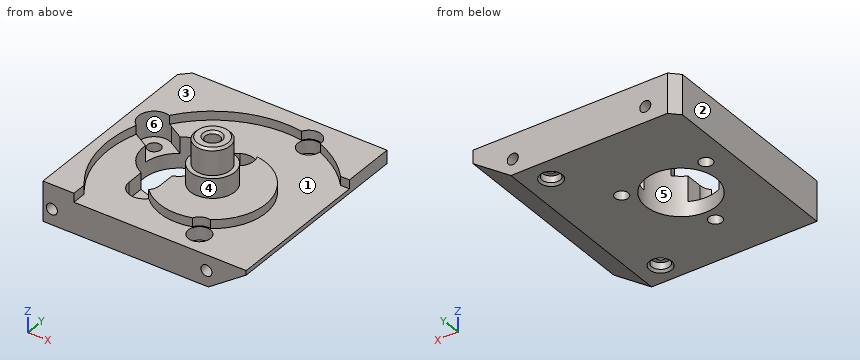
from build123d import *

# Parameters (mm, degrees)
SKETCH_1_W                  = 52
SKETCH_1_H                  = 47
EXTRUDE_1_DEPTH             = 9
SKETCH_19_R                 = 23.75
SKETCH_19_R_2               = 12
CUT_EXTRUDE_2_DEPTH         = 2
SKETCH_20_R                 = 5
EXTRUDE_3_DEPTH             = 4.4
SKETCH_21_R                 = 4
EXTRUDE_4_DEPTH             = 6
SKETCH_22_R                 = 8
CUT_EXTRUDE_5_DEPTH         = 37.556941885
CUT_EXTRUDE_6_DEPTH         = 47
HOLE_WIZARD_M3_1_D          = 2.5
HOLE_WIZARD_M3_1_DEPTH      = 9.5
HOLE_WIZARD_M3_1_TIP        = 0.751075774
HOLE_WIZARD_M4_2_D          = 3.3
HOLE_WIZARD_M4_2_DEPTH      = 10.1
HOLE_WIZARD_M4_2_TIP        = 0.991420021
CHAMFER_3_SIZE              = 0.5
CHAMFER_5_SIZE              = 2
EXTRUDE3_DEPTH              = 2
EXTRUDE4_REACH              = 57.474
CUT_EXTRUDE_START           = -31
SKETCH_34_R                 = 8
CUT_EXTRUDE_1_DEPTH         = 31
SKETCH_35_R                 = 3.25
CUT_EXTRUDE_2_2_DEPTH       = 33
PATTERN_CIRCULAR_1_COUNT    = 3
HOLE_WIZARD_2_AT_2_COUNT    = 2
HOLE_WIZARD_2_AT_2_PITCH    = 19.052558883
HOLE_WIZARD_2_AT_3_COUNT    = 2
HOLE_WIZARD_2_AT_3_PITCH    = 19.052558883
HOLE_WIZARD_M3_2_D          = 2.5
HOLE_WIZARD_M3_2_DEPTH      = 9.5
HOLE_WIZARD_M3_2_TIP        = 0.751075774
SKETCH_39_R                 = 2
CUT_EXTRUDE_3_DEPTH         = 2
SKETCH_40_R                 = 2.75
CUT_EXTRUDE_4_DEPTH         = 2
SKETCH_41_R                 = 1.1
CUT_EXTRUDE_5_2_DEPTH       = 37
CHAMFER_7_SIZE              = 0.5
HOLE_WIZARD_2_2_D           = 2
HOLE_WIZARD_2_2_CBORE_D     = 5
HOLE_WIZARD_2_2_CBORE_DEPTH = 3
CUT_EXTRUDE_START_2         = 7
CUT_EXTRUDE_7_DEPTH         = 7
PATTERN_CIRCULAR_2_COUNT    = 3
SKETCH_45_W                 = 2.943459277
SKETCH_45_H                 = 3.25
SKETCH_45_W_2               = 2.005209087
SKETCH_45_H_2               = 2.691311543
SKETCH_45_W_3               = 3.943459277
SKETCH_45_H_3               = 4.763787499
CUT_EXTRUDE_8_DEPTH         = 2


with BuildPart() as part:
    # 草图1 → 拉伸1 (new body)
    with BuildSketch(Plane.XY):
        Rectangle(SKETCH_1_W, SKETCH_1_H)
    extrude(amount=EXTRUDE_1_DEPTH)

    # 草图19 → Cut-Extrude 2 (cut)
    with BuildSketch(Plane.XY.offset(9)):
        with Locations((0, -4)):
            Circle(SKETCH_19_R)
        with Locations((0, -4)):
            Circle(SKETCH_19_R_2, mode=Mode.SUBTRACT)
    extrude(amount=-CUT_EXTRUDE_2_DEPTH, mode=Mode.SUBTRACT)

    # 草图20 → 拉伸3 (add)
    with BuildSketch(Plane.XY.offset(9)):
        with Locations((0, -4)):
            Circle(SKETCH_20_R)
    extrude(amount=EXTRUDE_3_DEPTH)

    # 草图21 → 拉伸4 (add)
    with BuildSketch(Plane.XY.offset(13.4)):
        with Locations((0, -4)):
            Circle(SKETCH_21_R)
    extrude(amount=EXTRUDE_4_DEPTH)

    # 草图22 → Cut-Extrude 5 (cut, through all)
    with BuildSketch(Plane.XY.offset(9)):
        with Locations((-11, 0.795831523)):
            Circle(SKETCH_22_R)
    extrude(amount=-CUT_EXTRUDE_5_DEPTH, mode=Mode.SUBTRACT)

    # 草图25 → 拉伸6 (cut)
    with BuildSketch(Plane.XZ.offset(23.5)):
        Polygon((26, 8), (14.574815946, 0), (26, 0), align=None)
    extrude(amount=-CUT_EXTRUDE_6_DEPTH, mode=Mode.SUBTRACT)

    # M3 螺纹孔1
    with Locations(Plane(origin=(11, 23.5, 3.5), x_dir=(0, 0, 1), z_dir=(0, 1, 0))):
        with Locations((0, 0), (0, -30)):
            Hole(HOLE_WIZARD_M3_1_D / 2, depth=HOLE_WIZARD_M3_1_DEPTH)
            with Locations((0, 0, -(HOLE_WIZARD_M3_1_DEPTH + HOLE_WIZARD_M3_1_TIP / 2))):  # 118° drill point
                Cone(0, HOLE_WIZARD_M3_1_D / 2, HOLE_WIZARD_M3_1_TIP, mode=Mode.SUBTRACT)

    # M4 螺纹孔2
    with Locations(Plane(origin=(0, -4, 19.4), x_dir=(1, 0, 0), z_dir=(0, 0, 1))):
        with Locations((0, 0)):
            Hole(HOLE_WIZARD_M4_2_D / 2, depth=HOLE_WIZARD_M4_2_DEPTH)
            with Locations((0, 0, -(HOLE_WIZARD_M4_2_DEPTH + HOLE_WIZARD_M4_2_TIP / 2))):  # 118° drill point
                Cone(0, HOLE_WIZARD_M4_2_D / 2, HOLE_WIZARD_M4_2_TIP, mode=Mode.SUBTRACT)

    # 倒角3
    chamfer_3_edges = [part.edges().sort_by_distance(p)[0] for p in [
        (-4, -4, 19.4),
        (1.65, -4, 19.4),
    ]]
    chamfer(chamfer_3_edges, length=CHAMFER_3_SIZE)

    # 倒角5
    chamfer_5_edges = [part.edges().sort_by_distance(p)[0] for p in [
        (-26, 23.5, 4.5),
    ]]
    chamfer(chamfer_5_edges, length=CHAMFER_5_SIZE)

    # Sketch4 → Extrude3 (cut)
    with BuildSketch(Plane.XZ.offset(23.5)):
        Polygon((-26, 0), (14.574815946, 0), (26, 8), (26, 9), (13.557746863, 9), (13.557746863, 7), (-13.557746863, 7), (-13.557746863, 9), (-26, 9), align=None)
    extrude(amount=-EXTRUDE3_DEPTH, mode=Mode.SUBTRACT)

    # Extrude4: up to this face of the body (flat: up to its plane)
    extrude4_end = Plane(part.part.faces().sort_by_distance((-1.330613504, 23.5, 4.737278788))[0])
    # Sketch5 → Extrude4 (cut, up to the picked face)
    with BuildSketch(Plane.XZ.offset(21.5), mode=Mode.PRIVATE) as extrude4_sk1:
        Polygon((26, 9), (20, 9), (20, 6), (11.43111196, 0), (14.574815946, 0), (26, 8), align=None)
    extrude4_tool1 = split(extrude(extrude4_sk1.sketch, amount=-EXTRUDE4_REACH, mode=Mode.PRIVATE), bisect_by=extrude4_end, keep=Keep.BOTH, mode=Mode.PRIVATE)
    add(extrude4_tool1.solids().sort_by(Axis((19.659359, -21.5, 5.073959), (0, 1, 0)))[0], mode=Mode.SUBTRACT)

    # 草图34 → 切除-拉伸1 (cut)
    with BuildSketch(Plane(origin=(0, 0, 0), x_dir=(-1, 0, 0), z_dir=(0, 0, -1)).offset(CUT_EXTRUDE_START)):
        with Locations(Location((11, 0.795831523, 0), (0, 0, 180))):
            Circle(SKETCH_34_R)
    extrude(amount=CUT_EXTRUDE_1_DEPTH, mode=Mode.SUBTRACT)

    # 草图35 → Cut-Extrude 2 2 (cut)
    with BuildSketch(Plane.XY.offset(7)):
        with Locations((-1.473720558, 6.295831523)):
            Circle(SKETCH_35_R)
    cut_extrude_2_2 = extrude(amount=CUT_EXTRUDE_2_2_DEPTH, mode=Mode.SUBTRACT)

    # 阵列(圆周)1: Cut-Extrude 2 2 ×3 about axis
    pattern_circular_1_axis = Axis((-11, 0.795831523, 0), (0, 0, 1))
    for i in range(1, PATTERN_CIRCULAR_1_COUNT):
        add(cut_extrude_2_2.rotate(pattern_circular_1_axis, i * 360 / PATTERN_CIRCULAR_1_COUNT), mode=Mode.SUBTRACT)

    # 草图36 → Hole Wizard 2 (revolve, cut)
    with BuildSketch(Plane(origin=(-20.526279442, 6.295831523, 7), x_dir=(0, -1, 0), z_dir=(1, 0, 0))):
        Polygon((0, 0), (0, 7), (1.5, 7), (1.5, 3.7), (3.5, 3.7), (3.5, 0), align=None)
    hole_wizard_2 = revolve(axis=Axis((-20.526279442, 6.295831523, 13.35), (0, 0, -1)), mode=Mode.SUBTRACT)

    # Hole Wizard 2 at 2: Hole Wizard 2 ×2
    with Locations(*[(i * HOLE_WIZARD_2_AT_2_PITCH, 0, 0) for i in range(1, HOLE_WIZARD_2_AT_2_COUNT)]):
        add(hole_wizard_2, mode=Mode.SUBTRACT)

    # Hole Wizard 2 at 3: Hole Wizard 2 ×2
    with Locations(*[Vector(0.49999999999999795, -0.8660254037844398, 0) * (i * HOLE_WIZARD_2_AT_3_PITCH) for i in range(1, HOLE_WIZARD_2_AT_3_COUNT)]):
        add(hole_wizard_2, mode=Mode.SUBTRACT)

    # M3 螺纹孔2
    with Locations(Plane(origin=(-24, -21.5, 3.5), x_dir=(0, 0, -1), z_dir=(0, -1, 0))):
        with Locations((0, 0), (0, 35)):
            Hole(HOLE_WIZARD_M3_2_D / 2, depth=HOLE_WIZARD_M3_2_DEPTH)
            with Locations((0, 0, -(HOLE_WIZARD_M3_2_DEPTH + HOLE_WIZARD_M3_2_TIP / 2))):  # 118° drill point
                Cone(0, HOLE_WIZARD_M3_2_D / 2, HOLE_WIZARD_M3_2_TIP, mode=Mode.SUBTRACT)

    # 草图39 → 切除-拉伸3 (cut)
    with BuildSketch(Plane(origin=(0, 0, 0), x_dir=(-1, 0, 0), z_dir=(0, 0, -1))):
        with Locations((-6, 18.295831523)):
            Circle(SKETCH_39_R)
        with Locations((-6, -16.704168477)):
            Circle(SKETCH_39_R)
    extrude(amount=-CUT_EXTRUDE_3_DEPTH, mode=Mode.SUBTRACT)

    # 草图40 → 切除-拉伸4 (cut)
    with BuildSketch(Plane.XY.offset(9)):
        with Locations((6, 18.295831523)):
            Circle(SKETCH_40_R)
        with Locations((6, -16.704168477)):
            Circle(SKETCH_40_R)
    extrude(amount=-CUT_EXTRUDE_4_DEPTH, mode=Mode.SUBTRACT)

    # 草图41 → Cut-Extrude 5 2 (cut)
    with BuildSketch(Plane(origin=(0, 0, 2), x_dir=(-1, 0, 0), z_dir=(0, 0, -1))):
        with Locations((-6, 18.295831523)):
            Circle(SKETCH_41_R)
        with Locations((-6, -16.704168477)):
            Circle(SKETCH_41_R)
    extrude(amount=-CUT_EXTRUDE_5_2_DEPTH, mode=Mode.SUBTRACT)

    # 倒角7
    chamfer_7_edges = [part.edges().sort_by_distance(p)[0] for p in [
        (8, 18.295831523, 0),
        (8, -16.704168477, 0),
    ]]
    chamfer(chamfer_7_edges, length=CHAMFER_7_SIZE)

    # Hole Wizard 2 2 (through all)
    with Locations(Plane(origin=(6, 18.295831523, 7), x_dir=(1, 0, 0), z_dir=(0, 0, 1))):
        with Locations((0, 0), (0, -35)):
            CounterBoreHole(HOLE_WIZARD_2_2_D / 2, HOLE_WIZARD_2_2_CBORE_D / 2, HOLE_WIZARD_2_2_CBORE_DEPTH)

    # 草图44 → 切除-拉伸7 (cut)
    with BuildSketch(Plane.XY.offset(3.3).offset(CUT_EXTRUDE_START_2)):
        with BuildLine():
            Line((0.276279442, 3.26474261), (-9.25, -2.23525739))
            ThreePointArc((-9.25, -2.23525739), (-14.031088913, -0.954168477), (-12.75, 3.826920437))
            Line((-12.75, 3.826920437), (-3.223720558, 9.326920437))
            ThreePointArc((-3.223720558, 9.326920437), (1.557368355, 8.045831523), (0.276279442, 3.26474261))
        make_face()
    cut_extrude_7 = extrude(amount=-CUT_EXTRUDE_7_DEPTH, mode=Mode.SUBTRACT)

    # 阵列(圆周)2: 切除-拉伸7 ×3 about axis
    pattern_circular_2_axis = Axis((-11, 0.795831523, 0), (0, 0, 1))
    for i in range(1, PATTERN_CIRCULAR_2_COUNT):
        add(cut_extrude_7.rotate(pattern_circular_2_axis, i * 360 / PATTERN_CIRCULAR_2_COUNT), mode=Mode.SUBTRACT)

    # 草图45 → 切除-拉伸8 (cut)
    with BuildSketch(Plane.XY.offset(9)):
        with Locations((-17.528270361, -19.875)):
            Rectangle(SKETCH_45_W, SKETCH_45_H)
        with Locations((18.997395457, 10.154344229)):
            Rectangle(SKETCH_45_W_2, SKETCH_45_H_2)
        with Locations((18.028270361, -19.11810625)):
            Rectangle(SKETCH_45_W_3, SKETCH_45_H_3)
    extrude(amount=-CUT_EXTRUDE_8_DEPTH, mode=Mode.SUBTRACT)


solid = part.part
Design review of the part built by this model. Coordinates are the model's own, in mm. Face numbers are marked on the shaded views. A direction names the side the tool comes from. Coordinates: 2 decimals unless noted, no trailing zeros. Loops run counter-clockwise (first coordinate to the right, second up) from the corner with the lowest first, then second, coordinate; pieces in that order, holes last.
Item 1: Clearance check with flat-ended pins moving along their axes: pin 1 (2.5 mm diameter, centred on x = 7, y = -18, fed in from +Z); pin 2 (1.5 mm diameter, centred on y = -5.5, z = 10, fed in from +X); pin 3 (2.5 mm diameter, centred on x = 6, y = -16.7, fed in from -Z). State where each tip first meets the part, or that it passes through.
Completed:
pin 1: stops at z = 7
pin 2: stops at x = 4.94
pin 3: stops at z = 2
Item 2: Add section B-B (x = -11). Write out the cut boundary in (y, z).
Completed:
outline: (-21.5, 0) - (-11.7, 0) - (-11.7, 3.3) - (-13.7, 3.3) - (-13.7, 7) - (-21.5, 7) - close; (-8.7, 0) - (-7.2, 0) - (-7.2, 3.3) - (-8.7, 3.3) - close; (8.8, 0) - (23.5, 0) - (23.5, 9) - (17.05, 9) - (17.05, 7) - (8.8, 7) - close
Item 3: Wall thickness on L1, parallel to Y at x = 6, z = 4.6; L2, parallel to Y at x = 6, z = 0.85; L3, parallel to Z at x = 11, y = -16: over which ranges is each line inside the solid? List them lowest first.
Completed:
L1: y = -21.5 to -19.2, -14.2 to 15.8, 20.8 to 23.5
L2: y = -21.5 to -18.7, -14.7 to 16.3, 20.3 to 23.5
L3: z = 0 to 2.25, 4.75 to 7
Item 4: Add section C-C (z = 18.25). Write out the cut boundary in (x, y).
Completed:
outline: circle Ø8 at (0, -4); hole circle Ø3.3 at (0, -4)
Item 5: For the marked faces 5 and 6, list the 3-axis set-ups (+Z, -Z, +X, -X, +Y, -Y) from which the entire face can be reached by the end or side of a thin tool; tool diameter is ignored.
Completed:
face 5: +Z, -Z
face 6: +Z
Item 6: Draft analysis for pull direction X (two halves, no side actions). For the marked faces 1, 2, 3 and 4, state which applies: pulls with the +X half, pulls with the -X half, needs draft (parallel to the pull), parting line crosses it, or undercut.
Completed:
face 1: undercut
face 2: pulls with the -X half
face 3: needs draft
face 4: parting line crosses it
Item 7: Add section D-D (x = 6). Give the number of separate pieces and of enclosed holes in the cut face, and give its area (3 significant figures).
Completed:
separate pieces: 3
enclosed holes: 0
area: 305 mm2
Item 8: Add section A-A (y = 6). Write out the cut boundary in (x, z).
Completed:
outline: (-26, 0) - (-22, 0) - (-22, 3.3) - (-24.01, 3.3) - (-24.01, 9) - (-26, 9) - close; (-19.06, 0) - (-17.08, 0) - (-17.08, 3.3) - (-19.06, 3.3) - close; (-4.92, 0) - (-2.94, 0) - (-2.94, 3.3) - (-4.92, 3.3) - close; (0, 0) - (11.43, 0) - (20, 6) - (20, 7) - (6.63, 7) - (6.63, 9) - (2.01, 9) - (2.01, 3.3) - (0, 3.3) - close
